from build123d import *

# Parameters (mm, degrees)
SALIENTE_EXTRUIR1_DEPTH = 7.9375


with BuildPart() as part:
    # Croquis1 → Saliente-Extruir1 (new body)
    with BuildSketch(Plane(origin=(0, 0, 0), x_dir=(1, 0, 0), z_dir=(0, 1, 0))):
        Polygon((70, -100), (0, -100), (0, 100), (70, 100), (185, 38.1), (185, -38.1), align=None)
        with BuildLine():
            ThreePointArc((41.5, -65), (35, -58.5), (28.5, -65))
            Line((28.5, -65), (28.5, -85))
            ThreePointArc((28.5, -85), (35, -91.5), (41.5, -85))
            Line((41.5, -85), (41.5, -65))
        make_face(mode=Mode.SUBTRACT)
        with BuildLine():
            ThreePointArc((160, -7.597922996), (167.597922996, 0), (160, 7.597922996))
            Line((160, 7.597922996), (100, 7.597922996))
            ThreePointArc((100, 7.597922996), (92.402077004, 0), (100, -7.597922996))
            Line((100, -7.597922996), (160, -7.597922996))
        make_face(mode=Mode.SUBTRACT)
        with BuildLine():
            Line((41.5, 85), (41.5, 65))
            ThreePointArc((41.5, 65), (35, 58.5), (28.5, 65))
            Line((28.5, 65), (28.5, 85))
            ThreePointArc((28.5, 85), (35, 91.5), (41.5, 85))
        make_face(mode=Mode.SUBTRACT)
    extrude(amount=SALIENTE_EXTRUIR1_DEPTH)


solid = part.part
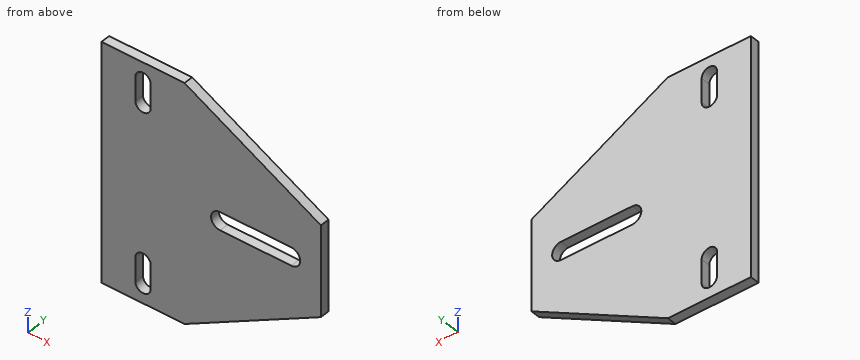
Part model, mm, in its own coordinate system. Give positions to 0.01 mm unless a question says otherwise; leave off trailing zeros. Order: outer loops, then holes, each group sorted by start corner. A loop starts at its lowest first (then second) coordinate and runs counter-clockwise, first axis right, second up. Notation, with made-up numbers: (53, -22.5) - (73, -22.5) arc R25 ccw to (73, -8.5) - close; hole circle Ø1 at (74, 27.25). An arc over 180 degrees is marked (long way). Use a Markdown table: item, result.
1) Probe L1, parallel to X at y = 5.75, z = 71; L2, parallel to Z at x = 37.5, y = 3.25; L3, parallel to X at y = 5.75, z = 87. List the from-to ranges inside material, lowest first. Write a range as from..to.
Checked values:
| item | result |
|---|---|
| L1 | 0..28.5, 41.5..123.88 |
| L2 | -100..-91, -59..59, 91..100 |
| L3 | 0..28.82, 41.18..94.15 |
2) Flat gauge pins, fed straight in: P1, Ø2, axis at x = 141, y = 1.5, coming from the +Z side; P2, Ø4, axis at x = 155, y = 4, coming from the -Z side; P3, Ø2.5, axis at x = 131.5, y = 2.5, coming from the +Z side. Where does each tip first touch, or does it go through?
Checked values:
| item | result |
|---|---|
| P1 | z = 62.32 |
| P2 | z = -55.32 |
| P3 | z = 67.57 |
3) Saw through at A-A on z = 0. List the corners of the cut face in (x, y).
Checked values:
| item | result |
|---|---|
| outline | (0, 0) - (92.4, 0) - (92.4, 7.94) - (0, 7.94) - close; (167.6, 0) - (185, 0) - (185, 7.94) - (167.6, 7.94) - close |
4) Saw through at D-D on z = 43. List the corners of the cut face in (x, y), plus the area to 3 significant figures.
Checked values:
| item | result |
|---|---|
| outline | (0, 0) - (175.9, 0) - (175.9, 7.94) - (0, 7.94) - close |
| area | 1,400 mm² |
5) Saw through at C-C on x = 147. List the corners of the cut face in (y, z).
Checked values:
| item | result |
|---|---|
| outline | (0, -58.55) - (7.94, -58.55) - (7.94, -7.6) - (0, -7.6) - close; (0, 7.6) - (7.94, 7.6) - (7.94, 58.55) - (0, 58.55) - close |
6) Saw through at B-B on y = 4. List the corners of the cut face in (x, z).
Checked values:
| item | result |
|---|---|
| outline | (0, -100) - (70, -100) - (185, -38.1) - (185, 38.1) - (70, 100) - (0, 100) - close; hole (28.5, -85) arc R6.5 ccw to (41.5, -85) - (41.5, -65) arc R6.5 ccw to (28.5, -65) - close; hole (28.5, 65) arc R6.5 ccw to (41.5, 65) - (41.5, 85) arc R6.5 ccw to (28.5, 85) - close; hole (100, -7.6) - (160, -7.6) arc R7.6 ccw to (160, 7.6) - (100, 7.6) arc R7.6 ccw to start |
